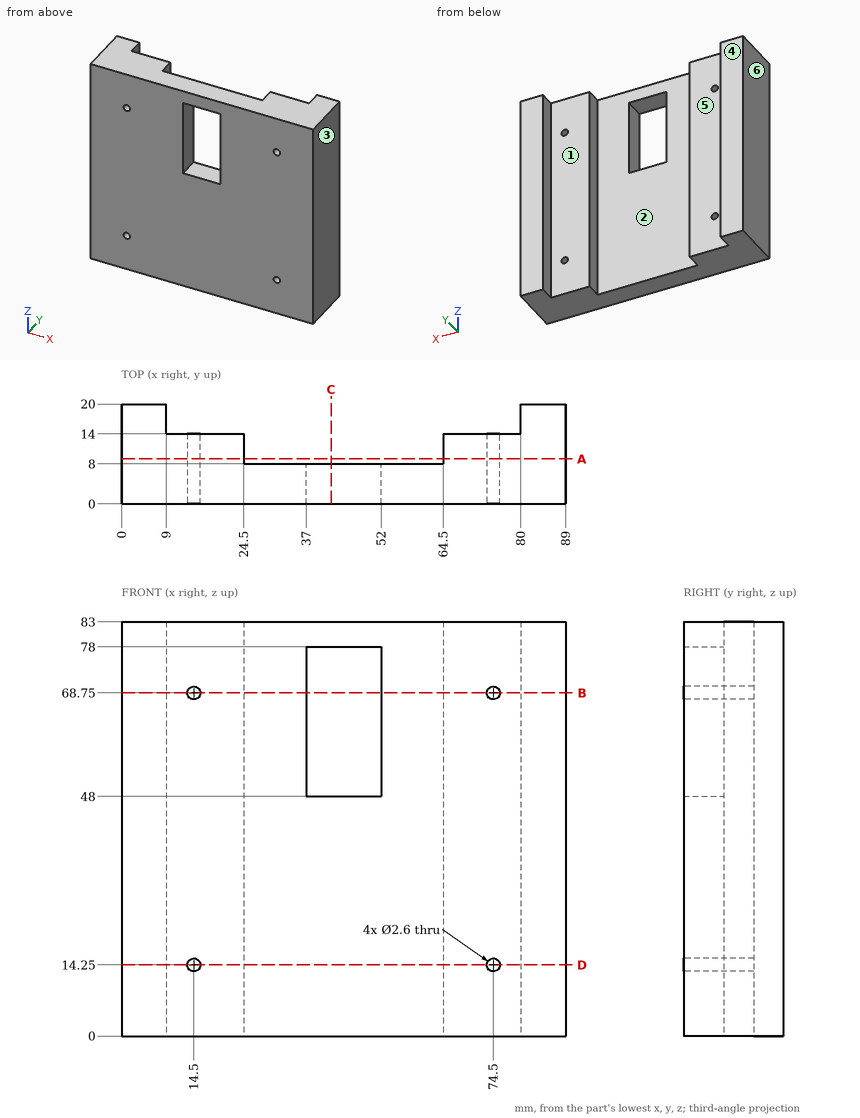
Answer from the drawing. Dimensions are ordinates in mm from the lowest x, y and z of the part. A direction names the side the tool comes from. Round coordinates to 2 decimals unless told otherwise and drop trailing zeros. Loops run counter-clockwise (first coordinate to the right, second up) from the corner with the lowest first, then second, coordinate; pieces in that order, holes last. Notation, with made-up numbers: (-10, 65) - (19, 65) arc R35 ccw to (19, 101) - close; hole circle Ø4 at (9.25, 56). An arc over 180 degrees is marked (long way). Return JSON: item names as keys, results as strings. Group by question number.
1. The part is cut by section D-D on z = 14.25. Determine the outline of the cut face in (x, y), then the cut area to 3 significant figures.
2. Which of the six approach directions +Z, -Z, +X, -X, +Y, -Y give full straight-line access (tool end or side, diameter ignored) to the marked faces 5 and 6?
3. Consider probe 1 along Z at (x, y) = (14.5, 3); probe 2 along X at (y, z) = (6.5, 14.25); probe 3 along X at (y, z) = (11, 14.25). Determine where each line is inside the solid, lowest interval first.
4. The part is cut by section C-C on x = 42. Determine the outline of the cut face in (y, z).
5. The part is cut by section B-B on z = 68.75. Determine the outline of the cut face in (x, y), then the cut area to 3 significant figures.
6. The mould has two halves that part along X. Classify the marked faces 1, 2, 3 and 4: pulls with the +X half, pulls with the -X half, needs draft (parallel to the pull), parting line crosses it, or undercut.
7. The part is cut by section A-A on y = 9. Determine the outline of the cut face in (x, z).
8. Each of these flat-tipped pins is pushed along its axis until it touches: P1, Ø8, axis at x = 15, z = 58, coming from the +Y side; P2, Ø10, axis at x = 56.5, z = 39, coming from the +Y side. Where does it stop, or does it pass through?
Resolved:
{
 "1": {"outline": "(0, 0) - (13.2, 0) - (13.2, 14) - (9, 14) - (9, 20) - (0, 20) - close; (15.8, 0) - (73.2, 0) - (73.2, 14) - (64.5, 14) - (64.5, 8) - (24.5, 8) - (24.5, 14) - (15.8, 14) - close; (75.8, 0) - (89, 0) - (89, 20) - (80, 20) - (80, 14) - (75.8, 14) - close", "area": "1,040 mm²"},
 "2": {"face 5": "+Z, -Z, +Y", "face 6": "+Z, -Z, -X, +Y, -Y"},
 "3": {"probe 1": "z = 0 to 12.95, 15.55 to 67.45, 70.05 to 83", "probe 2": "x = 0 to 13.2, 15.8 to 73.2, 75.8 to 89", "probe 3": "x = 0 to 13.2, 15.8 to 24.5, 64.5 to 73.2, 75.8 to 89"},
 "4": {"outline": "(0, 0) - (8, 0) - (8, 48) - (0, 48) - close; (0, 78) - (8, 78) - (8, 83) - (0, 83) - close"},
 "5": {"outline": "(0, 0) - (13.2, 0) - (13.2, 14) - (9, 14) - (9, 20) - (0, 20) - close; (15.8, 0) - (37, 0) - (37, 8) - (24.5, 8) - (24.5, 14) - (15.8, 14) - close; (52, 0) - (73.2, 0) - (73.2, 14) - (64.5, 14) - (64.5, 8) - (52, 8) - close; (75.8, 0) - (89, 0) - (89, 20) - (80, 20) - (80, 14) - (75.8, 14) - close", "area": "921 mm²"},
 "6": {"face 1": "undercut", "face 2": "undercut", "face 3": "pulls with the +X half", "face 4": "needs draft"},
 "7": {"outline": "(0, 0) - (24.5, 0) - (24.5, 83) - (0, 83) - close; (64.5, 0) - (89, 0) - (89, 83) - (64.5, 83) - close; hole circle Ø2.6 at (14.5, 14.25); hole circle Ø2.6 at (14.5, 68.75); hole circle Ø2.6 at (74.5, 14.25); hole circle Ø2.6 at (74.5, 68.75)"},
 "8": {"P1": "stops at y = 14", "P2": "stops at y = 8"}
}
